The listing builds one solid part. Answer for the finished solid, in the listing's coordinates (mm). A direction names the side the tool comes from. Coordinates: 2 decimals unless noted, no trailing zeros. Use one line per item in the form item = value. Start each with the question number.
Item 1: A tool of negligible diameter and unlimited length cuts with its end or side. For faces 1 (the cylindrical face through (-13.42, 5.7, -11.92)), 2 (the cylindrical face through (-7.952, 4.115, -12.751)), from which of +Z, -Z, +X, -X, +Y, -Y can it reach the whole face along a straight path? Write none if from no direction.
Item 2: Each of these flat-tipped pins is pushed along its axis until it touches: pin 1 Ø3 at (y, z) = (4.5, -4) entering from -X; pin 2 Ø3 at (x, y) = (-5.5, 3.5) entering from -Z; pin 3 Ø2 at (x, z) = (-3.5, -7) entering from -Y. Where does it stop, or does it pass through?
Item 3: Consider line 1 along Z through (x, y) = (-0.25, 3.3); line 2 along Z through (x, y) = (-10.25, 4.2); line 3 along Y through (x, z) = (-7.5, -7). Determine where each line is inside the solid, lowest interval first. Write a range as [from, to].
Item 4: The mould has two halves that part along Z. Classify faces 3 (the flat face through (-6, 3.682, -5)), 4 (the cylindrical face through (-0.97, 1.82, -1.27)), 5 (the flat face through (-5.511, 1.829, -0.566)), 6 (the cylindrical face through (-4.97, 1.83, -7.64)): released by +Z, released by -Z, zero draft, split by the parting line, or undercut.
Item 5: Section A-A, the plane y = 1.45 is taken. Count the separate pieces of the cut face and the enclosed holes in it, and give its area (3 significant figures).
from build123d import *

# Parameters (mm, degrees)
SKETCH1_R           = 1.6000000000000019
SKETCH1_R_2         = 1.6
BOSS_EXTRUDE1_DEPTH = 6
FILLET2_R           = 1
CUT_EXTRUDE1_START  = -2.3175
SKETCH3_R           = 1.6
CUT_EXTRUDE1_DEPTH  = 2.3175
FILLET3_R           = 1
FILLET4_R           = 1


with BuildPart() as part:
    # Sketch1 → Boss-Extrude1 (new body)
    with BuildSketch(Plane(origin=(0, 0, 0), x_dir=(1, 0, 0), z_dir=(0, 1, 0))):
        with BuildLine():
            Line((-14.129644992635422, 12.695385617697283), (-9.976148994946639, 4.396395245283378))
            ThreePointArc((-9.976148994946639, 4.396395245283378), (-9.61073090700793, 3.833838918319386), (-9.129445521149016, 3.3665441747595697))
            Line((-9.129445521149016, 3.3665441747595697), (-1.790159058231558, -2.3132132513522183))
            ThreePointArc((-1.790159058231558, -2.3132132513522183), (2.313213251352219, -1.790159058231561), (1.790159058231562, 2.3132132513522174))
            Line((1.790159058231562, 2.3132132513522174), (-4.4947536043408105, 7.1770075109265346))
            ThreePointArc((-4.4947536043408105, 7.1770075109265346), (-4.976038990199725, 7.644302254486349), (-5.3414570781384345, 8.20685858145034))
            Line((-5.3414570781384345, 8.20685858145034), (-8.898255102266939, 15.313602532880296))
            ThreePointArc((-8.898255102266939, 15.313602532880296), (-12.823058505042685, 16.62018902047303), (-14.129644992635422, 12.695385617697283))
        make_face()
        with Locations(Location((-11.51395004745118, 14.00449407528879, 0), (0, 0, 270))):
            Circle(SKETCH1_R, mode=Mode.SUBTRACT)
        with Locations(Location((1.73e-15, -8.7e-16, 0), (0, 0, 270))):
            Circle(SKETCH1_R_2, mode=Mode.SUBTRACT)
    extrude(amount=BOSS_EXTRUDE1_DEPTH)

    # Fillet2
    fillet2_edges = [part.edges().sort_by_distance(p)[0] for p in [
        (-12.05289699379103, 0, -8.545890431490331),
        (-12.823058505042688, 0, -16.62018902047303),
        (-7.119856090202687, 0, -11.760230557165318),
        (-4.976038990199726, 0, -7.64430225448635),
        (-12.823058505042688, 6, -16.62018902047303),
        (-12.05289699379103, 6, -8.545890431490331),
        (-9.61073090700793, 6, -3.833838918319386),
        (-5.459802289690288, 6, -0.5266654617036757),
        (2.3132132513522197, 6, 1.7901590582315603),
        (-1.352297273054624, 6, -4.745110381139376),
        (-4.976038990199726, 6, -7.64430225448635),
        (-1.352297273054624, 0, -4.745110381139376),
        (-7.119856090202687, 6, -11.760230557165318),
        (2.3132132513522197, 0, 1.7901590582315603),
        (-5.459802289690288, 0, -0.5266654617036757),
        (-9.61073090700793, 0, -3.833838918319386),
    ]]
    fillet(fillet2_edges, radius=FILLET2_R)

    # Sketch3 → Cut-Extrude1 (cut)
    # profile 1 of 2: a face of its own
    with BuildSketch(Plane(origin=(0, 6, 0), x_dir=(1, 0, 0), z_dir=(0, 1, 0)).offset(CUT_EXTRUDE1_START)):
        with BuildLine():
            ThreePointArc((-5.106773795189211, 6.386165373712101), (-5.748487643001094, 7.009225031791857), (-6.2357117602527055, 7.75930013441051))
            Line((-6.235711760252705, 7.75930013441051), (-8.449834443261716, 12.183280039497655))
            Line((-8.449834443261715, 12.183280039497657), (-11.892714969401661, 10.460180018394306))
            Line((-11.89271496940166, 10.460180018394302), (-9.08189431283237, 4.843953692323209))
            ThreePointArc((-9.08189431283237, 4.84395369232321), (-8.838282254206565, 4.4689161410138825), (-8.517425330300622, 4.157386311974004))
            Line((-8.517425330300622, 4.157386311974004), (-1.1781388673831632, -1.5223711141377843))
            ThreePointArc((-1.1781388673831628, -1.522371114137784), (1.5223711141377851, -1.1781388673831652), (1.1781388673831665, 1.5223711141377825))
            Line((1.178138867383166, 1.5223711141377825), (-5.10677379518921, 6.386165373712102))
        make_face()
        with Locations(Location((1.73e-15, -8.7e-16, 0), (0, 0, 270))):
            Circle(SKETCH3_R, mode=Mode.SUBTRACT)
    # profile 2 of 2: a face of its own
    with BuildSketch(Plane(origin=(0, 6, 0), x_dir=(1, 0, 0), z_dir=(0, 1, 0)).offset(CUT_EXTRUDE1_START)):
        with BuildLine():
            Line((-8.449834443261716, 12.183280039497655), (-6.235711760252705, 7.75930013441051))
            ThreePointArc((-6.2357117602527055, 7.75930013441051), (-5.748487643001094, 7.009225031791857), (-5.106773795189211, 6.386165373712101))
            Line((-5.10677379518921, 6.386165373712102), (1.178138867383166, 1.5223711141377825))
            ThreePointArc((1.1781388673831665, 1.5223711141377825), (1.5223711141377851, -1.1781388673831652), (-1.1781388673831628, -1.522371114137784))
            Line((-1.1781388673831632, -1.5223711141377843), (-8.517425330300622, 4.157386311974004))
            ThreePointArc((-8.517425330300622, 4.157386311974004), (-8.838282254206565, 4.4689161410138825), (-9.08189431283237, 4.84395369232321))
            Line((-9.08189431283237, 4.843953692323209), (-11.89271496940166, 10.460180018394302))
            Line((-11.892714969401661, 10.460180018394306), (-12.78696965151593, 10.012621571354474))
            Line((-12.78696965151593, 10.012621571354474), (-9.976148994946639, 4.396395245283378))
            ThreePointArc((-9.976148994946639, 4.396395245283378), (-9.61073090700793, 3.8338389183193877), (-9.129445521149018, 3.3665441747595706))
            Line((-9.129445521149016, 3.3665441747595715), (-1.790159058231558, -2.3132132513522183))
            ThreePointArc((-1.7901590582315579, -2.313213251352218), (2.3132132513522183, -1.7901590582315614), (1.7901590582315636, 2.3132132513522152))
            Line((1.7901590582315636, 2.313213251352215), (-4.4947536043408105, 7.1770075109265346))
            ThreePointArc((-4.4947536043408105, 7.177007510926534), (-4.976038990199726, 7.64430225448635), (-5.3414570781384345, 8.20685858145034))
            Line((-5.3414570781384345, 8.20685858145034), (-7.555579761147449, 12.630838486537487))
            Line((-7.555579761147449, 12.630838486537487), (-8.449834443261715, 12.183280039497657))
        make_face()
    extrude(amount=CUT_EXTRUDE1_DEPTH, mode=Mode.SUBTRACT)

    # Fillet3
    fillet3_edges = [part.edges().sort_by_distance(p)[0] for p in [
        (-6.448518419642942, 3.6825, -10.418848533993913),
        (-4.976038990199726, 3.6825, -7.64430225448635),
        (-1.3522972730546234, 3.6825, -4.745110381139375),
        (-5.459802289690288, 3.6825, -0.5266654617036766),
        (-11.381559323231285, 3.6825, -7.204508408318926),
        (-9.61073090700793, 3.6825, -3.8338389183193873),
        (2.3132132513522183, 3.6825, 1.7901590582315612),
    ]]
    fillet(fillet3_edges, radius=FILLET3_R)

    # Fillet4
    fillet4_edges = [part.edges().sort_by_distance(p)[0] for p in [
        (-12.525048519232481, 5.707106781186548, -10.14370840551512),
        (-10.171274706331689, 6, -11.32173002894598),
        (-7.817500893430897, 5.707106781186548, -12.49975165237684),
        (-12.786969651515932, 3.84125, -10.012621571354474),
        (-7.555579761147449, 3.84125, -12.630838486537488),
    ]]
    fillet(fillet4_edges, radius=FILLET4_R)


solid = part.part
Response:
q1.face_1 = +Z, -X, +Y
q1.face_2 = +X, +Y
q2.pin_1 = -10
q2.pin_2 = -11.23
q2.pin_3 = 0.12
q3.line_1 = [-3.62, -1.58], [1.58, 2.7]
q3.line_2 = [-16.64, -14.99], [-13.02, -11.28]
q3.line_3 = [0, 3.68]
q4.face_3 = zero draft
q4.face_4 = undercut
q4.face_5 = released by +Z
q4.face_6 = released by -Z
q5.separate_pieces = 1
q5.enclosed_holes = 2
q5.area = 120 mm2
